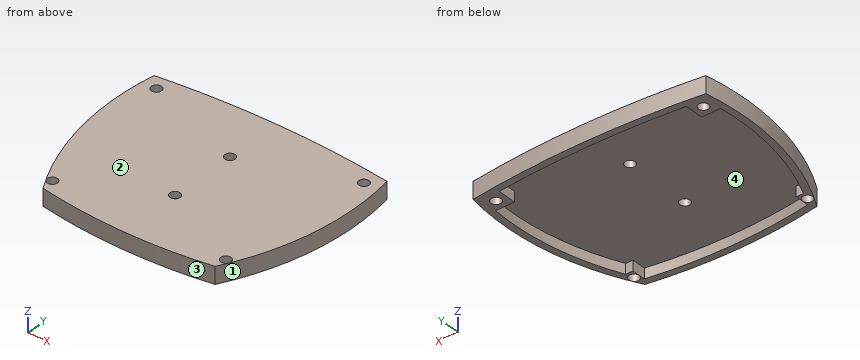
Autodesk Inventor part; units mm, degrees
ref_plane "YZ Plane" through (0, 0, 0) normal (1, 0, 0) x (0, 1, 0)
ref_plane "XZ Plane" through (0, 0, 0) normal (0, 1, 0) x (-1, 0, 0)
ref_plane "XY Plane" through (0, 0, 0) normal (0, 0, 1) x (1, 0, 0)
sketch "Sketch1" plane through (0, 0, 0) normal (0, 0, 1) x (1, 0, 0)
  line L0 (0, 0) -> (0, 23)
  line L1 (0, 0) -> (0, -25)
  line L2 (0, 0) -> (-32.5, 0)
  line L3 (0, 0) -> (32.5, 0)
  line L4 (0, 23) -> (0, 25)
  line L5 (0, -25) -> (0, -27)
  arc A0 (32.5, 23) -> (-32.5, 23) centre (0, -240.0625) ccw
  arc A1 (-24, -25) -> (24, -25) centre (0, 118) ccw
  arc A2 (-34.2324, 24.7969) -> (-25.28, -26.8099) centre (42.3382, 11.5) ccw
  arc A3 (34.2324, 24.7969) -> (-34.2324, 24.7969) centre (0, -240.0625) ccw
  arc A4 (25.28, -26.8099) -> (34.2324, 24.7969) centre (-42.3382, 11.5) ccw
  arc A5 (-25.28, -26.8099) -> (25.28, -26.8099) centre (0, 118) ccw
  line L6 (24, -25) -> (-24, -25)
  line L7 (-32.5, 23) -> (-30.5, 23)
  line L8 (-30.5, 23) -> (-30.5, 21)
  circle A6 centre (-30.5, 21) radius 1.5
  line L9 (-27.5, 23) -> (-27.5, 18)
  line L10 (-27.5, 18) -> (-33.0989, 18)
  line L11 (-32.5, 23) -> (-30.5, 23)
  line L12 (-27.5, 23) -> (27.5, 23)
  line L13 (-27.5, 23) -> (-27.5, 23.5696)
  circle A7 centre (30.5, 21) radius 1.5
  line L14 (27.5, 23) -> (27.5, 18)
  line L15 (27.5, 18) -> (33.0989, 18)
  line L16 (27.5, 23) -> (27.5, 23.5696)
  line L17 (-25.28, -26.8099) -> (-27.252, -26.8099)
  line L18 (-27.252, -26.8099) -> (-27.2519, -23.0989)
  line L19 (-27.2519, -23.0989) -> (-25.5309, -23.099)
  circle A8 centre (-25.5309, -23.099) radius 1.5
  line L20 (-26.1342, -20.8192) -> (-24, -20.8192)
  line L21 (-24, -20.8192) -> (-24, -25)
  arc A9 (-32.5, 23) -> (-26.1342, -20.8192) centre (42.3382, 11.5) ccw
  circle A10 centre (25.5309, -23.099) radius 1.5
  line L22 (26.1342, -20.8192) -> (24, -20.8192)
  line L23 (24, -20.8192) -> (24, -25)
  arc A11 (26.1342, -20.8192) -> (32.5, 23) centre (-42.3382, 11.5) ccw
  point P0 (24, -25)
  dimension "d0" = 23
  dimension "d1" = 25
  dimension "d4" = 65
  dimension "d6" = 48
  dimension "d7" = 32.5
  dimension "d8" = 32.5
  dimension "d9" = 2
  dimension "d10" = 2
  dimension "d12" = 2
  dimension "d13" = 2
  dimension "d14" = 3
  dimension "d15" = 5
  dimension "d16" = 5
  dimension "d17" = 1.972
  dimension "d18" = 3.711
  dimension "d19" = 1.721
  dimension "d20" = 3
extrude "Extrusion1" add sketch "Sketch1" along normal blind 2 contours L2 A9 L10 L9 L12 L0 | L3 A11 L22 L23 L6 L1 | L1 L6 L21 L20 A9 L2 | L0 L12 L14 L15 A11 L3 | L12 L13 A0 L4 | L4 A0 L16 L12 | L6 A1 L5 | L5 A1 L6 | A6 | L9 L10 A9 A0 L13 | L16 A0 A11 L15 L14 | A8 | A3 A4 A5 A2 | A7 | A10
extrude "Extrusion2" add sketch "Sketch1" against normal blind 3 contours L9 L10 A9 A0 L13 | L16 A0 A11 L15 L14 | A3 A4 A5 A2
sketch "Sketch2" plane through (0, 0, 2) normal (0, 0, 1) x (1, 0, 0)
  circle A0 centre (0, 10) radius 1.5
  circle A1 centre (0, -10) radius 1.5
  point P0 (0, 0)
  dimension "d27" = 3
  dimension "d28" = 3
extrude "Extrusion3" cut sketch "Sketch2" against normal up to surface (2 mm away)
extrude "Extrusion4" cut sketch "Sketch1" along normal blind 10 contours A6 | A8 | A7 | A10
properties part number "ProjEnAble_Microbit_Cover"
Could you check a few things on this model? Use its own coordinates, in mm. Face numbers are marked on the shaded views. Give positions to 0.01 mm unless a question says otherwise; leave off trailing zeros. Write each loop counter-clockwise with the first axis right and the second up, starting at its lowest first coordinate (ties: lowest second). Pieces come first, ordered by that corner, then holes. Notation, with made-up numbers: (18.5, 87.25) - (47.5, 87.25) arc R15 ccw to (47.5, 105.25) - close; hole circle Ø4 at (51, -21.75). An arc over 180 degrees is marked (long way). One line per item, written item: value. Start each with the question number.
Item 1: Imagine slicing it at B-B, the plane x = -30.5. List the corners of the cut face in (y, z) for me, and give its area (3 significant figures).
Item 2: I'm going to push flat-ended pins straight in: pin 1 (1.5 mm diameter, centred on y = -22.5, z = -2, fed in from +X); pin 2 (1.8 mm diameter, centred on x = 0, y = 10, fed in from +Z); pin 3 (1.1 mm diameter, centred on x = -25, z = -2, fed in from +Y); pin 4 (0.9 mm diameter, centred on y = 21, z = -1.5, fed in from -X). Where does each tip first touch, or does it pass through?
Item 3: Imagine slicing it at A-A, the plane x = 0. List the corners of the cut face in (y, z) for me.
Item 4: Please list where these lines run through material, in increasing order: line 1 (Y direction, x = 0, z = 1.4); line 2 (Y direction, x = 1.5, z = -0.35); line 3 (X direction, y = 21, z = -0.15). Write a range as from..to.
Item 5: Imagine slicing it at C-C, the plane y = 10. List the corners of the cut face in (x, z) for me.
Item 6: If we mould it in two halves opening along X, with no side actions, what happens to the marked faces 1, 2, 3 and 4? For each: +X half, -X half, draft (parallel to the pull), parting line (faces both ways), or undercut.
Item 7: Imagine slicing it at D-D, the plane z = -1.05. List the corners of the cut face in (x, y) for me (1 decimal), and give its area (3 significant figures).
Geometry says:
1. outline: (-15.6, -3) - (-9.18, -3) - (-9.18, 0) - (18, 0) - (18, -3) - (19.5, -3) - (19.5, 2) - (-15.6, 2) - close; (22.5, -3) - (25.25, -3) - (25.25, 2) - (22.5, 2) - close
1. area: 108 mm^2
2. pin 1: x = 27.91
2. pin 2: through
2. pin 3: y = 25.88
2. pin 4: x = -34.85
3. outline: (-29, -3) - (-27, -3) - (-27, 0) - (-11.5, 0) - (-11.5, 2) - (-29, 2) - close; (-8.5, 0) - (8.5, 0) - (8.5, 2) - (-8.5, 2) - close; (11.5, 0) - (25, 0) - (25, -3) - (27, -3) - (27, 2) - (11.5, 2) - close
4. line 1: -29..-11.5, -8.5..8.5, 11.5..27
4. line 2: -28.99..-26.99, 25..27
4. line 3: -34.8..-32, -29..-27.5, 27.5..29, 32..34.8
5. outline: (-35.36, -3) - (-33.36, -3) - (-33.36, 0) - (-1.5, 0) - (-1.5, 2) - (-35.36, 2) - close; (1.5, 0) - (33.36, 0) - (33.36, -3) - (35.36, -3) - (35.36, 2) - (1.5, 2) - close
6. face 1: +X half
6. face 2: draft
6. face 3: parting line
6. face 4: undercut
7. outline: (-34.2, 24.8) arc R77.7 ccw to (-25.3, -26.8) arc R147 ccw to (25.3, -26.8) arc R77.7 ccw to (34.2, 24.8) arc R267.1 ccw to start; hole (-33.1, 18) arc R75.7 ccw to (-26.1, -20.8) - (-24, -20.8) - (-24, -25) arc R145 ccw to (24, -25) - (24, -20.8) - (26.1, -20.8) arc R75.7 ccw to (33.1, 18) - (27.5, 18) - (27.5, 23.6) arc R265.1 ccw to (-27.5, 23.6) - (-27.5, 18) - close; hole circle Ø3 at (-30.5, 21); hole circle Ø3 at (-25.5, -23.1); hole circle Ø3 at (25.5, -23.1); hole circle Ø3 at (30.5, 21)
7. area: 476 mm^2
